For this review, take the finished solid that the model builds, in its own axes (mm). A direction names the side the tool comes from. Give positions to 0.01 mm unless a question says otherwise; leave off trailing zeros. Write each loop counter-clockwise with the first axis right and the second up, starting at its lowest first coordinate (ties: lowest second). Pieces come first, ordered by that corner, then holes. Notation, with made-up numbers: (15, 60.25) -> (62, 60.25) arc R21 ccw to (62, 90.25) -> close; hole circle Ø1 at (73.5, 70). An arc over 180 degrees is marked (long way). Answer as CSV lines item,"result".
```python
from build123d import *

# Parameters (mm, degrees)
CUT_EXTRUDE1_DEPTH = 59.855755878
CIRPATTERN1_COUNT  = 4


with BuildPart() as part:
    # Sketch1 → Revolve1 (revolve)
    with BuildSketch(Plane.XY, mode=Mode.PRIVATE) as revolve1_sk:
        Polygon((-13, 38), (13, 38), (13, 35), (4, 33), (4, 20), (20, 15), (20, 12), (-20, 12), (-20, 15), (-4, 20), (-4, 33), (-13, 35), align=None)
    revolve(revolve1_sk.sketch.rotate(Axis((0, 0, 0), (1, 0, 0)), 90), axis=Axis((0, 0, 0), (1, 0, 0)))

    # Sketch2 → Cut-Extrude1 (cut, symmetric)
    with BuildSketch(Plane.ZY.offset(4)):
        with BuildLine():
            ThreePointArc((13.461538462, 24.551720556), (0, 28), (-13.461538462, 24.551720556))
            ThreePointArc((-13.461538462, 24.551720556), (-14.253694325, 21.836487769), (-11.538461538, 21.044331905))
            ThreePointArc((-11.538461538, 21.044331905), (0, 24), (11.538461538, 21.044331905))
            ThreePointArc((11.538461538, 21.044331905), (14.253694325, 21.836487769), (13.461538462, 24.551720556))
        make_face()
    cut_extrude1 = extrude(amount=CUT_EXTRUDE1_DEPTH, both=True, mode=Mode.SUBTRACT)

    # CirPattern1: Cut-Extrude1 ×4 about axis
    cirpattern1_axis = Axis((0, 0, 0), (1, 0, 0))
    for i in range(1, CIRPATTERN1_COUNT):
        add(cut_extrude1.rotate(cirpattern1_axis, i * 360 / CIRPATTERN1_COUNT), mode=Mode.SUBTRACT)


solid = part.part
```
Q1. Add section A-A (y = 0). State how many separate pieces and enclosed holes the cut face has, plus the area to 3 significant figures.
Answer block:
separate pieces,"4"
enclosed holes,"0"
area,"848 mm2"
Q2. Clearance check with flat-ended pins moving along their axes: pin 1 (8 mm diameter, centred on x = -13, y = 26, fed in from +Z); pin 2 (12 mm diameter, centred on x = 10.5, y = -30, fed in from +Z); pin 3 (5 mm diameter, centred on x = -4, y = -26, fed in from +Z); pin 4 (14.5 mm diameter, centred on y = 0, z = 0, fed in from -X). State where each tip first meets the part, or that it passes through.
Answer block:
pin 1,"stops at z = 30.98"
pin 2,"stops at z = 29.46"
pin 3,"stops at z = 29.86"
pin 4,"passes through"
Q3. Add section D-D (x = 10). Write out the cut boundary in (y, z) (3 decimals).
Answer block:
outline,"circle Ø76 at (0, 0); circle Ø36.25 at (0, 0); hole circle Ø68.667 at (0, 0); hole circle Ø24 at (0, 0)"
Q4. Add section B-B (x = -3). Write out the cut boundary in (y, z), plus the area to 3 significant figures.
Answer block:
outline,"circle Ø76 at (0, 0); hole (-24.55, -13.46) arc R2 ccw to (-21.04, -11.54) arc R24 cw to (-21.04, 11.54) arc R2 ccw to (-24.55, 13.46) arc R28 ccw to start; hole (-13.46, -24.55) arc R28 ccw to (13.46, -24.55) arc R2 ccw to (11.54, -21.04) arc R24 cw to (-11.54, -21.04) arc R2 ccw to start; hole (-13.46, 24.55) arc R2 ccw to (-11.54, 21.04) arc R24 cw to (11.54, 21.04) arc R2 ccw to (13.46, 24.55) arc R28 ccw to start; hole circle Ø24 at (0, 0); hole (21.04, -11.54) arc R2 ccw to (24.55, -13.46) arc R28 ccw to (24.55, 13.46) arc R2 ccw to (21.04, 11.54) arc R24 cw to start"
area,"3,620 mm2"
Q5. Draft analysis for pull direction Z (two halves, no side actions). For faces 4 (the cylindrical face through (0, 24, 0)), 5 (the flat face through (13, 31, 17)), state which applies: released by +Z, released by -Z, zero draft, split by the parting line, or undercut.
Answer block:
face 4,"undercut"
face 5,"zero draft"
Q6. To check wall thickness, follow probe 1 along Z at (x, y) = (-0.5, 3); probe 2 along Y at (x, z) = (-9.5, 11); probe 3 along Z at (x, y) = (3, 7). State the ranges of each line that lie inside material, in increasing order. Write a range as [from, to].
Answer block:
probe 1,"z = [-37.88, -27.84], [-23.81, -11.62], [11.62, 23.81], [27.84, 37.88]"
probe 2,"y = [-36.37, -32.41], [-14.6, -4.8], [4.8, 14.6], [32.41, 36.37]"
probe 3,"z = [-37.35, -27.11], [-22.96, -9.75], [9.75, 22.96], [27.11, 37.35]"
Q7. For faces 1 (the flat face through (-13, 31, -17)), 2 (the cylindrical face through (0, -24, 0)), 3 (the flat face through (-20, -10, 7)), list the 3-axis set-ups (+Z, -Z, +X, -X, +Y, -Y) from which the entire face can be reached by the end or side of a thin tool; tool diameter is ignored.
Answer block:
face 1,"-X"
face 2,"+X, -X"
face 3,"+Z, -Z, -X, +Y, -Y"
